from build123d import *

# Parameters (mm, degrees)
SKETCH1_W           = 77
SKETCH1_H           = 114
BOSS_EXTRUDE1_DEPTH = 10
SKETCH2_W           = 73
SKETCH2_H           = 109
CUT_EXTRUDE1_DEPTH  = 6
SKETCH3_W           = 59
SKETCH3_H           = 35
CUT_EXTRUDE2_DEPTH  = 6
FILLET1_R           = 5
FILLET2_R           = 5
FILLET3_R           = 2
FILLET4_R           = 2
SKETCH7_W           = 27
SKETCH7_H           = 5
CUT_EXTRUDE8_DEPTH  = 6
FILLET5_R           = 2
CUT_EXTRUDE9_DEPTH  = 10
FILLET6_R           = 2
FILLET7_R           = 1


with BuildPart() as part:
    # Sketch1 → Boss-Extrude1 (new body)
    with BuildSketch(Plane.XY):
        with Locations((38.5, 51.816921292)):
            Rectangle(SKETCH1_W, SKETCH1_H)
    extrude(amount=BOSS_EXTRUDE1_DEPTH)

    # Sketch2 → Cut-Extrude1 (cut)
    with BuildSketch(Plane.XY.offset(10)):
        with Locations((38.5, 52.316921292)):
            Rectangle(SKETCH2_W, SKETCH2_H)
    extrude(amount=-CUT_EXTRUDE1_DEPTH, mode=Mode.SUBTRACT)

    # Sketch3 → Cut-Extrude2 (cut)
    with BuildSketch(Plane.XY.offset(4)):
        with Locations((38.5, 81.316921292)):
            Rectangle(SKETCH3_W, SKETCH3_H)
    extrude(amount=-CUT_EXTRUDE2_DEPTH, mode=Mode.SUBTRACT)

    # Fillet1
    fillet1_edges = [part.edges().sort_by_distance(p)[0] for p in [
        (0, 108.816921292, 5),
        (77, 108.816921292, 5),
        (77, -5.183078708, 5),
        (0, -5.183078708, 5),
    ]]
    fillet(fillet1_edges, radius=FILLET1_R)

    # Fillet2
    fillet2_edges = [part.edges().sort_by_distance(p)[0] for p in [
        (38.5, -5.183078708, 0),
        (0, 51.816921292, 0),
        (38.5, 108.816921292, 0),
        (77, 51.816921292, 0),
        (75.535533906, 107.352455198, 0),
        (1.464466094, 107.352455198, 0),
        (75.535533906, -3.718612614, 0),
        (1.464466094, -3.718612614, 0),
    ]]
    fillet(fillet2_edges, radius=FILLET2_R)

    # Fillet3
    fillet3_edges = [part.edges().sort_by_distance(p)[0] for p in [
        (9, 63.816921292, 2),
        (9, 98.816921292, 2),
        (68, 98.816921292, 2),
        (68, 63.816921292, 2),
    ]]
    fillet(fillet3_edges, radius=FILLET3_R)

    # Fillet4
    fillet4_edges = [part.edges().sort_by_distance(p)[0] for p in [
        (2, -2.183078708, 7),
        (2, 106.816921292, 7),
        (75, 106.816921292, 7),
        (75, -2.183078708, 7),
    ]]
    fillet(fillet4_edges, radius=FILLET4_R)

    # Sketch7 → Cut-Extrude8 (cut)
    with BuildSketch(Plane.XZ.offset(5.183078708)):
        with Locations((38.5, 7.5)):
            Rectangle(SKETCH7_W, SKETCH7_H)
    extrude(amount=-CUT_EXTRUDE8_DEPTH, mode=Mode.SUBTRACT)

    # Fillet5
    fillet5_edges = [part.edges().sort_by_distance(p)[0] for p in [
        (52, -3.683078708, 5),
        (25, -3.683078708, 5),
    ]]
    fillet(fillet5_edges, radius=FILLET5_R)

    # Sketch8 → Cut-Extrude9 (cut)
    with BuildSketch(Plane(origin=(0, 0, 0), x_dir=(-1, 0, 0), z_dir=(0, 0, -1))):
        with BuildLine():
            Line((-56, 27.816921292), (-21, 27.816921292))
            ThreePointArc((-21, 27.816921292), (-16, 22.816921292), (-21, 17.816921292))
            Line((-21, 17.816921292), (-56, 17.816921292))
            ThreePointArc((-56, 17.816921292), (-61, 22.816921292), (-56, 27.816921292))
        make_face()
    extrude(amount=-CUT_EXTRUDE9_DEPTH, mode=Mode.SUBTRACT)

    # Fillet6
    fillet6_edges = [part.edges().sort_by_distance(p)[0] for p in [
        (61, 22.816921292, 0),
        (38.5, 17.816921292, 0),
        (16, 22.816921292, 0),
        (38.5, 27.816921292, 0),
    ]]
    fillet(fillet6_edges, radius=FILLET6_R)

    # Fillet7
    fillet7_edges = [part.edges().sort_by_distance(p)[0] for p in [
        (68, 81.316921292, 0),
        (38.5, 63.816921292, 0),
        (9, 81.316921292, 0),
        (38.5, 98.816921292, 0),
        (67.414213562, 64.402707729, 0),
        (9.585786438, 64.402707729, 0),
        (9.585786438, 98.231134854, 0),
        (67.414213562, 98.231134854, 0),
    ]]
    fillet(fillet7_edges, radius=FILLET7_R)


solid = part.part
Can you work these out from the model? Positions are in its coordinate system, mm. A direction names the side the tool comes from. Coordinates: 2 decimals unless noted, no trailing zeros. Write each loop counter-clockwise with the first axis right and the second up, starting at its lowest first coordinate (ties: lowest second). Pieces come first, ordered by that corner, then holes. Notation, with made-up numbers: (-3.5, 29) - (52.5, 29) arc R15 ccw to (52.5, 44) - close; hole circle Ø3 at (-0.5, 61). An arc over 180 degrees is marked (long way). Return JSON: item names as keys, results as strings. Group by question number.
Item 1: If we section it at A-A (x = 36): Write out the boundary of the cut face in (y, z).
Item 2: Which directions (+Z, -Z, +X, -X, +Y, -Y) give clear straight access to the entire face, cutting with the end or side of a thin tool? Please do faces 1 (the face through (38, 41, 4)), 2 (the face through (38.969, -3.68, 1.426)), 3 (the face through (38, 98.817, 3)), 4 (the face through (38, -4, 5)).
Item 3: We'd pull the mould along Y, two halves only. Please class faces 5 (the face through (1.426, -3.68, 7.535)), 6 (the face through (38, 63.817, 3)), 7 (the face through (1, 56, 10)): pulls with the +Y half, pulls with the -Y half, needs draft (parallel to the pull), parting line crosses it, or undercut.
Item 4: If we section it at D-D (z = 8.25): Write out the boundary of the cut face in (x, y).
Item 5: Please list where these lines run through material, in increasing order: probe 1 along Y at (x, z) = (69, 5.25); probe 2 along X at (y, z) = (62, 8); probe 3 along Y at (x, z) = (36, 1.25).
Item 6: If we section it at C-C (y = 9.5): Write out the boundary of the cut face in (x, z).
Item 7: I'm going to push flat-ended pins straight in: pin 1 Ø4 at (y, z) = (53, 2) entering from +X; pin 2 Ø2 at (x, z) = (13.5, 2.5) entering from -Y; pin 3 Ø3.5 at (x, z) = (26.5, 2.5) entering from +Y. Where does each tip first touch, or does it pass through?
Item 8: If we section it at B-B (y = 84.5): Write out the boundary of the cut face in (x, z), then the cut area to 3 significant figures.
Return value:
{
 "1": {"outline": "(-5.18, 5) arc R5 ccw to (-0.18, 0) - (15.82, 0) arc R2 ccw to (17.82, 2) - (17.82, 4) - (-2.18, 4) - (-2.18, 5) - close; (27.82, 2) arc R2 ccw to (29.82, 0) - (62.82, 0) arc R1 ccw to (63.82, 1) - (63.82, 4) - (27.82, 4) - close; (98.82, 1) arc R1 ccw to (99.82, 0) - (103.82, 0) arc R5 ccw to (108.82, 5) - (108.82, 10) - (106.82, 10) - (106.82, 4) - (98.82, 4) - close"},
 "2": {"face 1": "+Z", "face 2": "-Z, +X, -X, -Y", "face 3": "+Z, -Z", "face 4": "+Z, -Y"},
 "3": {"face 5": "pulls with the -Y half", "face 6": "undercut", "face 7": "needs draft"},
 "4": {"outline": "(0, -0.18) arc R5 ccw to (5, -5.18) - (25, -5.18) - (25, -2.18) - (4, -2.18) arc R2 cw to (2, -0.18) - (2, 104.82) arc R2 cw to (4, 106.82) - (73, 106.82) arc R2 cw to (75, 104.82) - (75, -0.18) arc R2 cw to (73, -2.18) - (52, -2.18) - (52, -5.18) - (72, -5.18) arc R5 ccw to (77, -0.18) - (77, 103.82) arc R5 ccw to (72, 108.82) - (5, 108.82) arc R5 ccw to (0, 103.82) - close"},
 "5": {"probe 1": "y = -5.18 to -2.18, 106.82 to 108.82", "probe 2": "x = 0 to 2, 75 to 77", "probe 3": "y = -3.49 to 17.67, 27.96 to 63.82, 98.82 to 107.12"},
 "6": {"outline": "(0, 5) arc R5 ccw to (5, 0) - (72, 0) arc R5 ccw to (77, 5) - (77, 10) - (75, 10) - (75, 4) - (2, 4) - (2, 10) - (0, 10) - close"},
 "7": {"pin 1": "stops at x = 76.9", "pin 2": "stops at y = -4.95", "pin 3": "stops at y = 108.76"},
 "8": {"outline": "(0, 5) arc R5 ccw to (5, 0) - (8, 0) arc R1 ccw to (9, 1) - (9, 4) - (2, 4) - (2, 10) - (0, 10) - close; (68, 1) arc R1 ccw to (69, 0) - (72, 0) arc R5 ccw to (77, 5) - (77, 10) - (75, 10) - (75, 4) - (68, 4) - close", "area": "84.8 mm^2"}
}
